Verification items for this drawing (mm, ordinates from the low corner). Coordinates: 2 decimals unless noted, no trailing zeros. Loops run counter-clockwise (first coordinate to the right, second up) from the corner with the lowest first, then second, coordinate; pieces in that order, holes last. Notation, with made-up numbers: M -22.75,-22 L 32.25,-22 A19 ccw 32.25,-10 Z; hole C -32.75,41.5 d6. An arc over 180 degrees is marked long. Return JSON: item names as keys, results as strings.
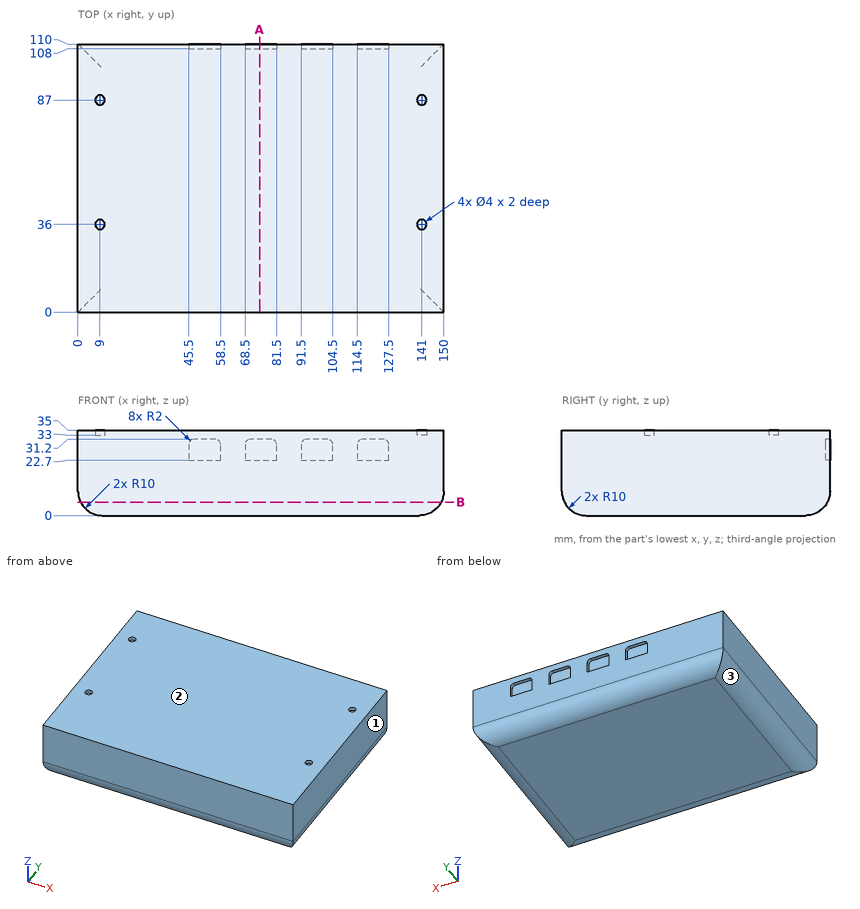
1) Draft check along X on the marked faces 1, 2 and 3. Enter one of: +X half, -X half, draft (parallel to the pull), parting line (faces both ways), or undercut.
Answers:
{"face 1": "+X half", "face 2": "draft", "face 3": "-X half"}
2) Section check A-A on x = 74.5. Record the cut outline in (y, z).
Answers:
{"outline": "M 0,10 A10 ccw 10,0 L 100,0 A10 ccw 110,10 L 110,22.7 L 108,22.7 L 108,31.2 L 110,31.2 L 110,35 L 0,35 Z"}
3) Section check B-B on z = 5.5. Record the cut outline in (x, y), then the cut area to 3 significant figures.
Answers:
{"outline": "M 1.07,1.07 L 148.93,1.07 L 148.93,108.93 L 1.07,108.93 Z", "area": "15,900 mm²"}
4) Scan lines: line 1 along Y through (x, z) = (9, 33.85); line 2 along Y through (x, z) = (47.5, 30); line 3 along Z through (x, y) = (144.5, 63). Record each from-to range of solid material in increasing order. Write a range as [from, to].
Answers:
{"line 1": "[0, 34], [38, 85], [89, 110]", "line 2": "[0, 108]", "line 3": "[1.07, 35]"}
5) Go/stop test with flat-tipped pins: pin 1 Ø6.5 at (x, y) = (9, 36) entering from -Z; pin 2 Ø1 at (x, y) = (77, 108.5) entering from -Z; pin 3 Ø1.2 at (x, y) = (140.5, 87) entering from +Z; pin 4 Ø1 at (x, z) = (56.5, 3.5) entering from +Y. Record where each tip stops, or that it passes through.
Answers:
{"pin 1": "z = 0", "pin 2": "z = 4", "pin 3": "z = 33", "pin 4": "y = 108"}
